```python
from build123d import *

# Parameters (mm, degrees)
SKETCH1_R           = 6.35
BOSS_EXTRUDE1_DEPTH = 6.35
SKETCH2_R           = 9.525
BOSS_EXTRUDE2_DEPTH = 3.175
SKETCH3_R           = 6.35
CUT_EXTRUDE1_DEPTH  = 43.709869791


with BuildPart() as part:
    # Sketch1 → Boss-Extrude1 (new body)
    with BuildSketch(Plane.XY):
        with BuildLine():
            Line((-30.746408046, 10.565086207), (20.053591954, 10.565086207))
            ThreePointArc((20.053591954, 10.565086207), (29.578591954, 1.040086207), (20.053591954, -8.484913793))
            Line((20.053591954, -8.484913793), (-30.746408046, -8.484913793))
            ThreePointArc((-30.746408046, -8.484913793), (-40.271408046, 1.040086207), (-30.746408046, 10.565086207))
        make_face()
        with Locations((-30.746408046, 1.040086207)):
            Circle(SKETCH1_R, mode=Mode.SUBTRACT)
        with Locations((20.053591954, 1.040086207)):
            Circle(SKETCH1_R, mode=Mode.SUBTRACT)
    extrude(amount=BOSS_EXTRUDE1_DEPTH)

    # Sketch2 → Boss-Extrude2 (add)
    with BuildSketch(Plane.XY.offset(6.35)):
        with Locations(Location((20.053591954, 1.040086207, 0), (0, 0, 90))):
            Circle(SKETCH2_R)
    extrude(amount=BOSS_EXTRUDE2_DEPTH)

    # Sketch3 → Cut-Extrude1 (cut, through all)
    with BuildSketch(Plane(origin=(0, 0, 0), x_dir=(-1, 0, 0), z_dir=(0, 0, -1))):
        with Locations((-20.053591954, 1.040086207)):
            Circle(SKETCH3_R)
    extrude(amount=-CUT_EXTRUDE1_DEPTH, mode=Mode.SUBTRACT)


solid = part.part
```
Here's how the part is built. I have some questions about the finished solid (model axes, mm). A direction names the side the tool comes from. Round coordinates to 2 decimals unless told otherwise and drop trailing zeros. Loops run counter-clockwise (first coordinate to the right, second up) from the corner with the lowest first, then second, coordinate; pieces in that order, holes last.
1. If I drill on probe 1 along X at (y, z) = (1, 6.25); probe 2 along X at (y, z) = (2.5, 6); probe 3 along Z at (x, y) = (-26, -3.5), over which ranges is the centre line in solid material (lowest first)?
Answers:
probe 1: x = -40.27 to -37.1, -24.4 to 13.7, 26.4 to 29.58
probe 2: x = -40.16 to -36.93, -24.57 to 13.87, 26.23 to 29.47
probe 3: z = 0 to 6.35
2. For faces 4 (the face through (-5, -8.485, 3)), 5 (the face through (29.352, -1.025, 5.754)), which set-ups out of +Z, -Z, +X, -X, +Y, -Y let a thin tool reach every point of the face, with its end or its side?
Answers:
face 4: +Z, -Z, +X, -X, -Y
face 5: +Z
3. Suppose I cut it at A-A, the plane x = 25. Please give me the cut outline in (y, z) (3 decimals), and give its area (3 significant figures).
Answers:
outline: (-7.1, 0) - (-2.942, 0) - (-2.942, 9.525) - (-7.1, 9.525) - close; (5.022, 0) - (9.18, 0) - (9.18, 9.525) - (5.022, 9.525) - close
area: 79.2 mm2
4. Will these pins go through, and if not, where does the flat tip stop? pin 1 (5 mm diameter, centred on y = 6.5, z = 3.5, fed in from -X); pin 2 (5 mm diameter, centred on x = -3.5, y = -5, fed in from -Z); pin 3 (6 mm diameter, centred on x = -10.5, y = -6.5, fed in from +Z); pin 4 (3 mm diameter, centred on x = 10.5, z = 8.5, fed in from +Y).
Answers:
pin 1: stops at x = -39.8
pin 2: stops at z = 0
pin 3: stops at z = 6.35
pin 4: stops at y = 6.13
5. Suppose I cut it at D-D, the plane z = 8.25. Please give me the cut outline in (x, y) (3 decimals), and give its area (3 significant figures).
Answers:
outline: circle Ø19.05 at (20.054, 1.04); hole circle Ø12.7 at (20.054, 1.04)
area: 158 mm2
6. Suppose I cut it at C-C, the plane y = -2.25. Please give me the cut outline in (x, z) (3 decimals).
Answers:
outline: (-39.685, 0) - (-36.178, 0) - (-36.178, 6.35) - (-39.685, 6.35) - close; (-25.315, 0) - (14.622, 0) - (14.622, 9.525) - (11.115, 9.525) - (11.115, 6.35) - (-25.315, 6.35) - close; (25.485, 0) - (28.992, 0) - (28.992, 9.525) - (25.485, 9.525) - close
7. Suppose I cut it at B-B, the plane y = 3.5. Please give me the cut outline in (x, z) (3 decimals), and give its area (3 significant figures).
Answers:
outline: (-39.948, 0) - (-36.601, 0) - (-36.601, 6.35) - (-39.948, 6.35) - close; (-24.892, 0) - (14.199, 0) - (14.199, 9.525) - (10.852, 9.525) - (10.852, 6.35) - (-24.892, 6.35) - close; (25.908, 0) - (29.255, 0) - (29.255, 9.525) - (25.908, 9.525) - close
area: 312 mm2
8. Thinking about a two-plate mould opening in X: for faces 1 (the face through (-40.27, 0.83, 3.13)), 2 (the face through (-5, 1, 0)), 3 (the face through (-37.09, 1.32, 3.13)), which applies, released by +X, released by -X, zero draft, split by the parting line, or undercut?
Answers:
face 1: released by -X
face 2: zero draft
face 3: undercut
